The listing builds one solid part. Answer for the finished solid, in the listing's coordinates (mm). Face numbers are marked on the shaded views. A direction names the side the tool comes from. Give positions to 0.01 mm unless a question says otherwise; leave off trailing zeros. Write each loop counter-clockwise with the first axis right and the second up, starting at its lowest first coordinate (ties: lowest second). Pieces come first, ordered by that corner, then holes. Notation, with made-up numbers: (42.5, -9) - (75.5, -9) arc R33 ccw to (75.5, 30) - close; hole circle Ø2 at (-29, 6). An arc over 180 degrees is marked (long way). One line per item, written item: value. Start each with the question number.
from build123d import *

# Parameters (mm, degrees)
SKETCH1_W           = 60
SKETCH1_H           = 218
BOSS_EXTRUDE1_DEPTH = 5
SKETCH2_W           = 50
SKETCH2_H           = 50
BOSS_EXTRUDE3_DEPTH = 2
LPATTERN1_COUNT     = 4
LPATTERN1_PITCH     = 52
SKETCH3_W           = 52
SKETCH3_H           = 51.9
BOSS_EXTRUDE8_DEPTH = 25
LPATTERN5_COUNT     = 4
LPATTERN5_PITCH     = 52


with BuildPart() as part:
    # Sketch1 → Boss-Extrude1 (new body)
    with BuildSketch(Plane(origin=(0, 0, 0), x_dir=(1, 0, 0), z_dir=(0, 1, 0))):
        Rectangle(SKETCH1_W, SKETCH1_H)
    extrude(amount=BOSS_EXTRUDE1_DEPTH)

    # Sketch2 → Boss-Extrude3 (add)
    with BuildSketch(Plane(origin=(0, 5, 0), x_dir=(1, 0, 0), z_dir=(0, 1, 0))):
        with Locations((0, -79)):
            Rectangle(SKETCH2_W, SKETCH2_H)
    boss_extrude3 = extrude(amount=BOSS_EXTRUDE3_DEPTH)

    # LPattern1: Boss-Extrude3 ×4
    with Locations(*[(0, 0, -i * LPATTERN1_PITCH) for i in range(1, LPATTERN1_COUNT)]):
        add(boss_extrude3)

    # Sketch3 → Boss-Extrude8 (add)
    with BuildSketch(Plane(origin=(0, 7, 0), x_dir=(1, 0, 0), z_dir=(0, 1, 0))):
        with Locations((0, -79.05)):
            Rectangle(SKETCH3_W, SKETCH3_H)
    boss_extrude8 = extrude(amount=BOSS_EXTRUDE8_DEPTH)

    # LPattern5: Boss-Extrude8 ×4
    with Locations(*[(0, 0, -i * LPATTERN5_PITCH) for i in range(1, LPATTERN5_COUNT)]):
        add(boss_extrude8)


solid = part.part
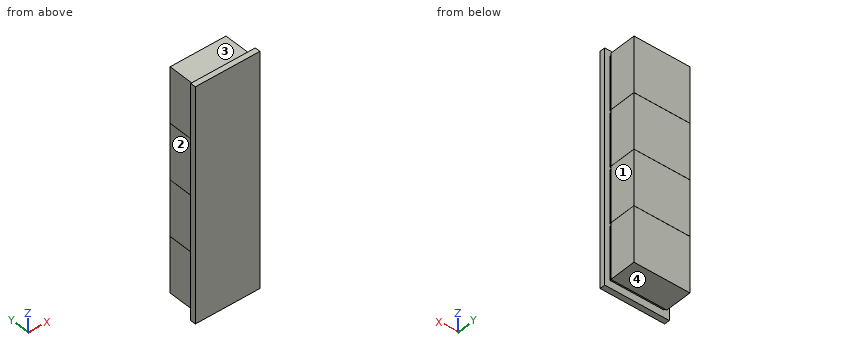
Item 1: Each of these flat-tipped pins is pushed along its axis until it touches: pin 1 Ø2 at (x, y) = (-9, 5.5) entering from -Z; pin 2 Ø1.6 at (x, y) = (-6.5, 6) entering from +Z; pin 3 Ø12.5 at (y, z) = (19.5, -80) entering from -X; pin 4 Ø2 at (x, y) = (-15.5, 20.5) entering from -Z. Where does it stop, or does it pass through?
Item 2: Straight lines are drawn through the part: line 1 along X through (y, z) = (7.5, 55); line 2 along Y through (x, z) = (26.5, 84). For each, find the intervals that lie inside material, in ascending order.
Item 3: Find section B-B on z = 50. Determine the outline of the cut face in (x, y), plus the area to 3 significant figures.
Item 4: Find section A-A on y = 9. Determine the outline of the cut face in (x, z).
Item 5: For the marked faces 1, 2, 3 and 4, determine the directions among +Z, -Z, +X, -X, +Y, -Y from which every point of the face is accessible in a straight line to the end or side of a thin tool.
Values:
1. pin 1: z = -109
1. pin 2: z = 104
1. pin 3: x = -26
1. pin 4: z = -102.9
2. line 1: -26 to 26
2. line 2: 0 to 5
3. outline: (-30, 0) - (30, 0) - (30, 5) - (25, 5) - (25, 7) - (26, 7) - (26, 32) - (-26, 32) - (-26, 7) - (-25, 7) - (-25, 5) - (-30, 5) - close
3. area: 1,700 mm^2
4. outline: (-26, -102.9) - (26, -102.9) - (26, -51) - (-26, -51) - close; (-26, -50.9) - (26, -50.9) - (26, 1) - (-26, 1) - close; (-26, 1.1) - (26, 1.1) - (26, 53) - (-26, 53) - close; (-26, 53.1) - (26, 53.1) - (26, 105) - (-26, 105) - close
5. face 1: +Z, -Z, +X, +Y
5. face 2: +Z, -Z, -X, +Y
5. face 3: +Z, +X, -X, +Y
5. face 4: -Z, +X, -X, +Y
